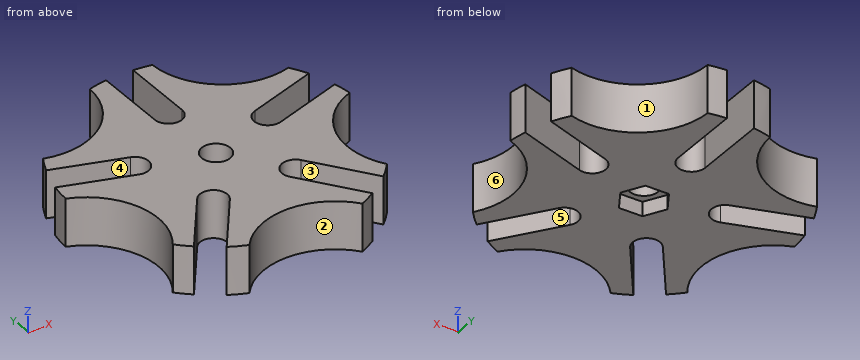
from build123d import *

# Parameters (mm, degrees)
MODEL_R                 = 3
BOSS_EXTRUDE3_DEPTH     = 10
CUT_EXTRUDE1_DEPTH      = 3
CUT_EXTRUDE1_DEPTH_BACK = 3


with BuildPart() as part:
    # Model → Boss-Extrude3 (new body)
    with BuildSketch(Plane.XY):
        with BuildLine():
            add(Edge.make_bspline(
                [(-27.783884398, 11.720720152), (-27.312273784, 12.880782387), (-26.795019787, 14.018174114), (-26.185754442, 15.108459083)],
                knots=[0.852290179, 0.852290179, 0.852290179, 0.852290179, 0.87243197, 0.87243197, 0.87243197, 0.87243197], degree=3))
            ThreePointArc((-26.185754442, 15.108459083), (-13.183686547, 17.45567821), (-7.081525862, 29.174331808))
            add(Edge.make_bspline(
                [(-7.081525862, 29.174331808), (-5.777480255, 29.53777265), (-4.469238519, 29.818781923), (-3.142641746, 29.977736074)],
                knots=[0, 0, 0, 0, 0.021616293, 0.021616293, 0.021616293, 0.021616293], degree=3))
            Line((-3.142641746, 29.977736074), (-3.047607508, 14.694279391))
            ThreePointArc((-3.047607508, 14.694279391), (-0.161689439, 11.892698747), (2.656409066, 14.762489335))
            Line((2.656409066, 14.762489335), (2.561374827, 30.045946018))
            add(Edge.make_bspline(
                [(2.561374827, 30.045946018), (3.81039527, 29.955896616), (5.051959359, 29.815432204), (6.277155329, 29.572903012)],
                knots=[0.052290179, 0.052290179, 0.052290179, 0.052290179, 0.07243197, 0.07243197, 0.07243197, 0.07243197], degree=3))
            ThreePointArc((6.277155329, 29.572903012), (12.527353316, 17.932532214), (25.558126537, 15.750295644))
            add(Edge.make_bspline(
                [(25.558126537, 15.750295644), (26.306751572, 14.62238397), (26.978276202, 13.465008783), (27.53939153, 12.252459811)],
                knots=[0.2, 0.2, 0.2, 0.2, 0.221616293, 0.221616293, 0.221616293, 0.221616293], degree=3))
            Line((27.53939153, 12.252459811), (13.033327655, 7.439229031))
            ThreePointArc((13.033327655, 7.439229031), (11.260663856, 3.828821816), (14.860837224, 2.035464932))
            Line((14.860837224, 2.035464932), (29.366901099, 6.848695711))
            add(Edge.make_bspline(
                [(29.366901099, 6.848695711), (29.667227572, 5.632979885), (29.91730238, 4.408776378), (30.065249788, 3.168600124)],
                knots=[0.252290179, 0.252290179, 0.252290179, 0.252290179, 0.27243197, 0.27243197, 0.27243197, 0.27243197], degree=3))
            ThreePointArc((30.065249788, 3.168600124), (20.926016685, -6.372763797), (22.87731675, -19.440113767))
            add(Edge.make_bspline(
                [(22.87731675, -19.440113767), (22.03594686, -20.50064236), (21.14273017, -21.496948837), (20.162921741, -22.405299465)],
                knots=[0.4, 0.4, 0.4, 0.4, 0.421616293, 0.421616293, 0.421616293, 0.421616293], degree=3))
            Line((20.162921741, -22.405299465), (11.102646985, -10.096582999))
            ThreePointArc((11.102646985, -10.096582999), (7.121162438, -9.526356728), (6.52809344, -13.504502824))
            Line((6.52809344, -13.504502824), (15.588368196, -25.81321929))
            add(Edge.make_bspline(
                [(15.588368196, -25.81321929), (14.524959722, -26.474523589), (13.437950364, -27.090658554), (12.30419092, -27.614600438)],
                knots=[0.452290179, 0.452290179, 0.452290179, 0.452290179, 0.47243197, 0.47243197, 0.47243197, 0.47243197], degree=3))
            ThreePointArc((12.30419092, -27.614600438), (0.405636244, -21.871116843), (-11.419167214, -27.764946697))
            add(Edge.make_bspline(
                [(-11.419167214, -27.764946697), (-12.687787438, -27.292477739), (-13.911350342, -26.750853818), (-15.078020581, -26.099696408)],
                knots=[0.6, 0.6, 0.6, 0.6, 0.621616293, 0.621616293, 0.621616293, 0.621616293], degree=3))
            Line((-15.078020581, -26.099696408), (-6.171514453, -13.679260495))
            ThreePointArc((-6.171514453, -13.679260495), (-6.85954343, -9.716434063), (-10.826253597, -10.381706678))
            Line((-10.826253597, -10.381706678), (-19.732759725, -22.802142592))
            add(Edge.make_bspline(
                [(-19.732759725, -22.802142592), (-20.690308779, -21.995135299), (-21.612192316, -21.151724141), (-22.460841595, -20.235361781)],
                knots=[0.652290179, 0.652290179, 0.652290179, 0.652290179, 0.67243197, 0.67243197, 0.67243197, 0.67243197], degree=3))
            ThreePointArc((-22.460841595, -20.235361781), (-20.675319699, -7.144329784), (-29.934750212, 2.280433012))
            add(Edge.make_bspline(
                [(-29.934750212, 2.280433012), (-29.877430739, 3.63296348), (-29.740417511, 4.964011949), (-29.481650943, 6.274799988)],
                knots=[0.8, 0.8, 0.8, 0.8, 0.821616293, 0.821616293, 0.821616293, 0.821616293], degree=3))
            Line((-29.481650943, 6.274799988), (-14.916852679, 1.642335072))
            ThreePointArc((-14.916852679, 1.642335072), (-11.360593424, 3.521270227), (-13.219086134, 7.088255236))
            Line((-13.219086134, 7.088255236), (-27.783884398, 11.720720152))
        make_face()
        Circle(MODEL_R, mode=Mode.SUBTRACT)
    extrude(amount=BOSS_EXTRUDE3_DEPTH)

    # Sketch2 → Cut-Extrude1 (cut, two sides)
    with BuildSketch(Plane.XY) as cut_extrude1_sk:
        Polygon((-2.402263966, 4.270729193), (-4.899691957, 0.054942975), (-2.497427991, -4.215786218), (2.402263966, -4.270729193), (4.899691957, -0.054942975), (2.497427991, 4.215786218), align=None)
    extrude(amount=CUT_EXTRUDE1_DEPTH, mode=Mode.SUBTRACT)
    extrude(cut_extrude1_sk.sketch, amount=-CUT_EXTRUDE1_DEPTH_BACK, mode=Mode.SUBTRACT)


solid = part.part
Model file for the job. Use its own axes, mm. Face numbers are marked on the shaded views. A direction names the side the tool comes from. Coordinates: 2 decimals unless noted, no trailing zeros. Write each loop counter-clockwise with the first axis right and the second up, starting at its lowest first coordinate (ties: lowest second). Pieces come first, ordered by that corner, then holes. Notation, with made-up numbers: (53, -4.75) - (79, -4.75) arc R6 cw to (79, -0.75) - close; hole circle Ø9 at (51.5, 12). An arc over 180 degrees is marked (long way). Write each question's results on one line, items separated by ' | '. Start each with the question number.
1) Cut at A-A (y = -24). Write the cut outline in (x, z), then the cut area to 3 significant figures.
2) Cut at C-C (y = -5.5). Write the cut outline in (x, z), then the cut area to 3 significant figures.
3) Probe line 1 along X through (y, z) = (-19, 1.75); line 2 along Y through (x, z) = (-14, 6.25); line 3 along Y through (x, z) = (0, 7.5). List the from-to ranges inside material, lowest first. Write a range as from..to.
4) Flat gauge pins, fed straight in: P1, Ø2, axis at x = -21, z = 7, coming from the +Y side; P2, Ø4, axis at y = 15.5, z = 4.5, coming from the +X side; P3, Ø5, axis at x = 0, y = 0, coming from the -Z side; P4, Ø2, axis at y = 15.5, z = 3.5, coming from the +X side. Where does each tip first touch, or does it go through?
5) 3-axis set-ups, long thin cutter, end or side, ignore diameter. For the marked faces 4, 5 and 6: which of +Z, -Z, +X, -X, +Y, -Y reach the whole face in a straight line?
6) Cut at B-B (x = 0). Write the cut outline in (y, z).
7) Mould opens along Y. For the marked faces 1, 2 and 3 say: pulls with the +Y half, pulls with the -Y half, needs draft (parallel to the pull), parting line crosses it, or undercut.
Returned:
1) outline: (-13.57, 0) - (-7.2, 0) - (-7.2, 10) - (-13.57, 10) - close; (8.2, 0) - (14.25, 0) - (14.25, 10) - (8.2, 10) - close | area: 124 mm^2
2) outline: (-21.33, 0) - (21.23, 0) - (21.23, 10) - (-21.33, 10) - close | area: 426 mm^2
3) line 1: -21.71..-17.01, -9.99..10.57, 17.66..22.58 | line 2: -26.66..-24.6, -14.81..1.52, 7.34..16.9 | line 3: -21.88..-3, 3..11.9
4) P1: y = 14.68 | P2: x = 26.91 | P3: through | P4: x = 26.35
5) face 4: +Z, -Z, -X | face 5: +Z, -Z | face 6: +Z, -Z, +X
6) outline: (-21.88, 0) - (-4.24, 0) - (-4.24, 3) - (-3, 3) - (-3, 10) - (-21.88, 10) - close; (3, 3) - (4.24, 3) - (4.24, 0) - (11.9, 0) - (11.9, 10) - (3, 10) - close
7) face 1: pulls with the +Y half | face 2: pulls with the -Y half | face 3: undercut
